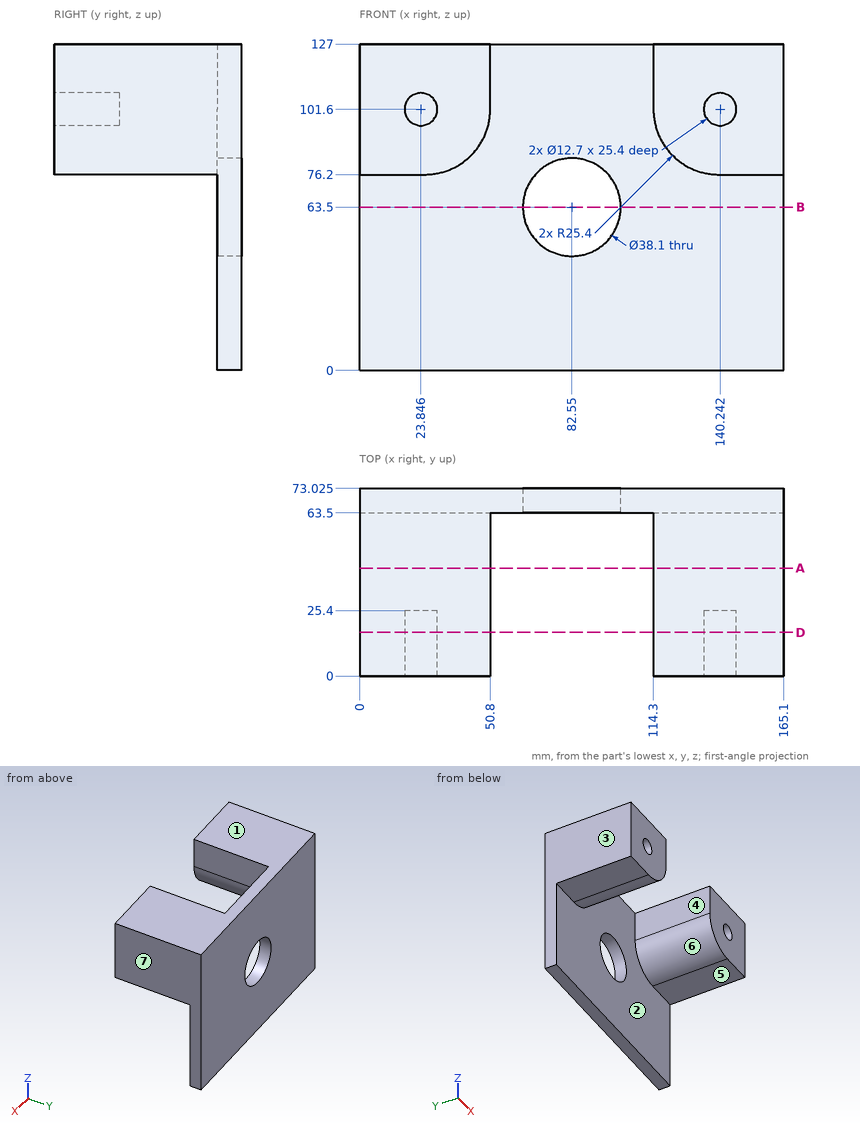
Verification items for this drawing (mm, ordinates from the low corner). A direction names the side the tool comes from. Give positions to 0.01 mm unless a question says otherwise; leave off trailing zeros. Loops run counter-clockwise (first coordinate to the right, second up) from the corner with the lowest first, then second, coordinate; pieces in that order, holes last. Notation, with made-up numbers: (44, 6.5) - (80, 6.5) arc R19 cw to (80, 28.5) - close; hole circle Ø7 at (50.25, 28). An arc over 180 degrees is marked (long way). Write item = value, one per line. Start each with the question number.
Q1. Tool access check on the marked faces 4, 5, 6 and 7. Record the directions out of +Z, -Z, +X, -X, +Y, -Y that give a thin tool (end or side, any length) a straight path to the whole face; none if there is none.
Q2. Mould release check, pull along X, two halves, no side actions. Record for the marked faces 1, 2 and 3: released by +X, released by -X, zero draft, split by the parting line, or undercut.
Q3. Cross-section at B-B, the plane z = 63.5. Enter the section's corners in (x, y) (1 decimal).
Q4. Depth check by flat-ended pin: P1, Ø7.5, axis at x = 7.5, y = 18, coming from the -Z side; P2, Ø8, axis at x = 113.5, z = 42.5, coming from the -Y side; P3, Ø10, axis at x = 108.5, y = 63, coming from the -Z side; P4, Ø6.5, axis at x = 22, z = 102.5, coming from the -Y side. Enter the tip coordinate at first touch or a pass-through.
Q5. Cross-section at D-D, the plane y = 17. State how many separate pieces and enclosed holes the cut face has, and give its area (3 significant figures).
Q6. Cross-section at A-A, the plane y = 42. Enter the section's corners in (x, z), and give its area (3 significant figures).
Q7. Thickness scan on line 1 (X direction, y = 3, z = 115); line 2 (X direction, y = 67, z = 63); line 3 (Y direction, x = 55.5, z = 8.5) (1 decimal). Record the ranges inside material, lowest first.
Answer key:
q1.face_4 = +Z, -Z, -Y
q1.face_5 = -Z, +X, -X, -Y
q1.face_6 = -Z, -Y
q1.face_7 = +Z, -Z, +X, +Y, -Y
q2.face_1 = zero draft
q2.face_2 = undercut
q2.face_3 = released by -X
q3.outline = (0, 63.5) - (63.5, 63.5) - (63.5, 73) - (0, 73) - close; (101.6, 63.5) - (165.1, 63.5) - (165.1, 73) - (101.6, 73) - close
q4.P1 = 76.2
q4.P2 = 63.5
q4.P3 = 0
q4.P4 = 25.4
q5.separate_pieces = 2
q5.enclosed_holes = 2
q5.area = 4,630 mm^2
q6.outline = (0, 76.2) - (25.4, 76.2) arc R25.4 ccw to (50.8, 101.6) - (50.8, 127) - (0, 127) - close; (114.3, 101.6) arc R25.4 ccw to (139.7, 76.2) - (165.1, 76.2) - (165.1, 127) - (114.3, 127) - close
q6.area = 4,880 mm^2
q7.line_1 = 0 to 50.8, 114.3 to 165.1
q7.line_2 = 0 to 63.51, 101.59 to 165.1
q7.line_3 = 63.5 to 73
